```python
from build123d import *

# Parameters (mm, degrees)
F2_R    = 5.08
F3_SIZE = 5.08
F4_SIZE = 0.254


with BuildPart() as f1:
    # F0 (on Front) → F1 (revolve)
    with BuildSketch(Plane.XZ):
        with BuildLine():
            Line((-95.25, 0), (0, 0))
            ThreePointArc((0, 0), (-2.708279, 3.647233), (-6.98284, 2.109309))
            ThreePointArc((-6.98284, 2.109309), (-8.264886, 7.499956), (-11.609642, 11.917572))
            ThreePointArc((-11.609642, 11.917572), (-11.088297, 14.546759), (-8.96451, 16.181984))
            Line((-8.96451, 16.181984), (-20.623778, 12.617388))
            ThreePointArc((-20.623778, 12.617388), (-30.0627, 10.566624), (-39.710517, 10.099176))
            Line((-39.710517, 10.099176), (-42.90622, 13.294879))
            Line((-42.90622, 13.294879), (-45.600297, 10.600802))
            ThreePointArc((-45.600297, 10.600802), (-57.823459, 13.638481), (-69.111465, 19.22544))
            Line((-69.111465, 19.22544), (-75.184, 21.082))
            Line((-75.184, 21.082), (-81.28, 21.082))
            Line((-81.28, 21.082), (-81.28, 31.75))
            Line((-81.28, 31.75), (-87.63, 31.75))
            Line((-87.63, 31.75), (-87.63, 44.45))
            Line((-87.63, 44.45), (-95.25, 44.45))
            Line((-95.25, 44.45), (-95.25, 0))
        make_face()
    revolve(axis=Axis((-47.625, 0, 0), (-1, 0, 0)))

    # F2
    f2_edges = [f1.edges().sort_by_distance(p)[0] for p in [
        (-87.63, 0, -44.45),
    ]]
    fillet(f2_edges, radius=F2_R)

    # F3
    f3_edges = [f1.edges().sort_by_distance(p)[0] for p in [
        (-81.28, 0, -31.75),
    ]]
    chamfer(f3_edges, length=F3_SIZE)

    # F4
    f4_edges = [f1.edges().sort_by_distance(p)[0] for p in [
        (-95.25, 0, -44.45),
        (-42.90622, 0, -13.294879),
    ]]
    chamfer(f4_edges, length=F4_SIZE)


solid = f1.part
```
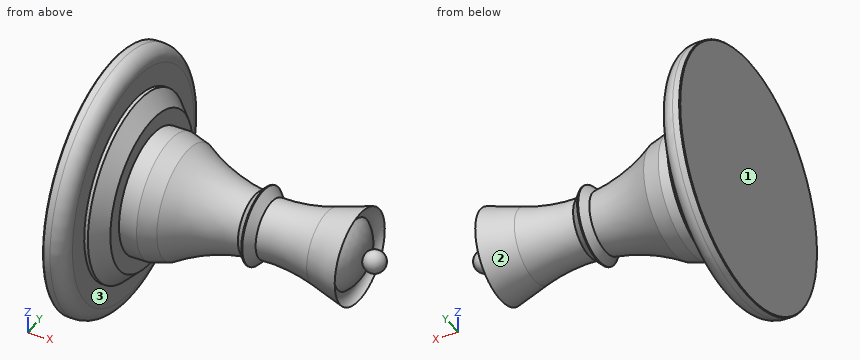
Check sheet for the modelled part. Datum: model origin and axes. Units: mm. Face numbers are marked on the shaded views. Give positions to 0.01 mm unless a question says otherwise; leave off trailing zeros. Order: outer loops, then holes, each group sorted by start corner. A loop starts at its lowest first (then second) coordinate and runs counter-clockwise, first axis right, second up. Notation, with made-up numbers: (30, 60) -> (48, 60) arc R25 cw to (48, 95) -> close; hole circle Ø5 at (4.5, 46). An arc over 180 degrees is marked (long way). Return JSON: item names as keys, results as strings.
1. Cross-section at B-B, the plane x = -67. Record the cut outline in (y, z).
From the geometry:
{"outline": "circle Ø35.88 at (0, 0)"}
2. Material ranges on probe 1 along X at (y, z) = (32, -15); probe 2 along X at (y, z) = (12.5, 20); probe 3 along Y at (x, z) = (-35, -2), recorded low to high. Write a range as [from, to].
From the geometry:
{"probe 1": "[-95.25, -87.63]", "probe 2": "[-95.25, -81.28]", "probe 3": "[-9.93, 9.93]"}
3. Cross-section at A-A, the plane x = -24. Record the cut outline in (y, z), plus the area to 3 significant figures.
From the geometry:
{"outline": "circle Ø23.39 at (0, 0)", "area": "430 mm^2"}
4. Mould release check, pull along X, two halves, no side actions. Record for the marked faces 1, 2 and 3: +X half, -X half, draft (parallel to the pull), parting line (faces both ways), or undercut.
From the geometry:
{"face 1": "-X half", "face 2": "undercut", "face 3": "+X half"}
5. Go/stop test with flat-tipped pins: P1, Ø8, axis at x = -65, y = 14.5, coming from the -Z side; P2, Ø12, axis at x = -28, z = -15.5, coming from the +Y side; P3, Ø10, axis at y = 31, z = -11.5, coming from the +X side. Record where each tip stops, or that it passes through.
From the geometry:
{"P1": "z = -14.27", "P2": "y = 5.52", "P3": "x = -82.67"}
